Design review of the part built by this model. Coordinates are the model's own, in mm. Face numbers are marked on the shaded views. A direction names the side the tool comes from. Coordinates: 2 decimals unless noted, no trailing zeros. Loops run counter-clockwise (first coordinate to the right, second up) from the corner with the lowest first, then second, coordinate; pieces in that order, holes last.
Q1. Wall thickness on probe 1 along Z at (x, y) = (-3, -1); probe 2 along Y at (x, z) = (3, 3); probe 3 along Z at (x, y) = (-2, -0.5): over which ranges is each line inside the solid? List them lowest first.
Q2. For P1, Ø1, axis at x = -2.5, y = -1.5, coming from the +Z side; P2, Ø1, axis at x = 2.5, y = -0.5, coming from the +Z side; P3, Ø1.5, axis at x = 0, z = 6.5, coming from the +Y side, all flat-tipped, find the tip position at first contact; note any pin that passes through.
Q3. Add section A-A on x = 0. Give the boundary of the cut face in (y, z).
Q4. Draft analysis for pull direction Z (two halves, no side actions). For the marked faces 1, 2 and 3, state which applies: released by +Z, released by -Z, zero draft, split by the parting line, or undercut.
Q5. Add section D-D on z = 7.25. Give the boundary of the cut face in (x, y), and give its area (3 significant figures).
Q6. Add section C-C on z = 5.75. Give the boundary of the cut face in (x, y).
Q7. Machinability: for the marked faces 4 and 5, which of the approach directions +Z, -Z, +X, -X, +Y, -Y give a long, thin tool a straight path to every point of the face, cutting with its end or side? Answer none if there is none.
```python
from build123d import *

# Parameters (mm, degrees)
F0_W    = 2
F0_H    = 1.75
F2_SIZE = 0.3


with BuildPart() as f1:
    # F0 (on Front) → F1 (revolve)
    with BuildSketch(Plane.XZ):
        Polygon((0, 5), (0, 0), (3.5, 0), (3.5, 5), (2, 5), align=None)
        with Locations((1, 5.875)):
            Rectangle(F0_W, F0_H)
        Polygon((0, 7.75), (0, 6.75), (2, 6.75), (2.1, 6.75), (2.1, 7.75), align=None)
    revolve(axis=Axis((0, 0, 2.5), (0, 0, 1)))

    # F2
    f2_edges = [f1.edges().sort_by_distance(p)[0] for p in [
        (-2.1, 0, 7.75),
        (-3.5, 0, 0),
    ]]
    chamfer(f2_edges, length=F2_SIZE)


solid = f1.part
```
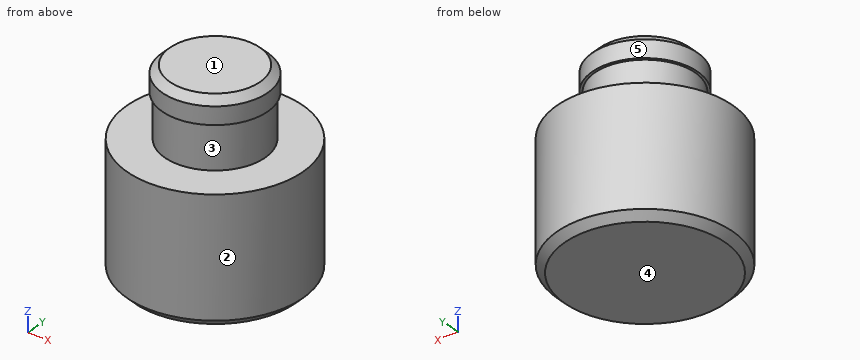
Entries:
1. probe 1: z = 0 to 5
1. probe 2: y = -1.8 to 1.8
1. probe 3: z = 0 to 5, 6.75 to 7.49
2. P1: stops at z = 5
2. P2: stops at z = 7.5
2. P3: stops at y = 2.1
3. outline: (-3.5, 0.3) - (-3.2, 0) - (3.2, 0) - (3.5, 0.3) - (3.5, 5) - (2, 5) - (2, 6.75) - (2.1, 6.75) - (2.1, 7.45) - (1.8, 7.75) - (-1.8, 7.75) - (-2.1, 7.45) - (-2.1, 6.75) - (-2, 6.75) - (-2, 5) - (-3.5, 5) - close
4. face 1: released by +Z
4. face 2: zero draft
4. face 3: undercut
5. outline: circle Ø4.2 at (0, 0)
5. area: 13.9 mm2
6. outline: circle Ø4 at (0, 0)
7. face 4: -Z, +X, -X, +Y, -Y
7. face 5: +Z
